from build123d import *

# Parameters (mm, degrees)
SKETCH1_W            = 20
SKETCH1_H            = 20
BOSS_EXTRUDE1_DEPTH  = 6.35
M5_CLEARANCE_HOLE1_D = 5.5
FILLET1_R            = 2.5


with BuildPart() as part:
    # Sketch1 → Boss-Extrude1 (new body)
    with BuildSketch(Plane(origin=(0, 0, 0), x_dir=(1, 0, 0), z_dir=(0, 1, 0))):
        Rectangle(SKETCH1_W, SKETCH1_H)
    extrude(amount=BOSS_EXTRUDE1_DEPTH)

    # M5 Clearance Hole1 (through all)
    with Locations(Plane(origin=(0, 6.35, 0), x_dir=(1, 0, 0), z_dir=(0, 1, 0))):
        with Locations((0, 0)):
            Hole(M5_CLEARANCE_HOLE1_D / 2)

    # Fillet1
    fillet1_edges = [part.edges().sort_by_distance(p)[0] for p in [
        (10, 3.175, 10),
        (-10, 3.175, 10),
        (-10, 3.175, -10),
        (10, 3.175, -10),
    ]]
    fillet(fillet1_edges, radius=FILLET1_R)


solid = part.part
Work out the finished part from the listing and answer in its coordinate system (mm). Coordinates: 2 decimals unless noted, no trailing zeros. Write each loop counter-clockwise with the first axis right and the second up, starting at its lowest first coordinate (ties: lowest second). Pieces come first, ordered by that corner, then holes. Notation, with made-up numbers: M -7.75,-13.75 L 50.25,-13.75 A12 ccw 50.25,-1.75 Z; hole C 32,56 d3. An arc over 180 degrees is marked long. Write item = value, one per line.
1. The part is cut by section B-B (y = 4.25). Determine the outline of the cut face in (x, z).
Solution:
outline = M -10,-7.5 A2.5 ccw -7.5,-10 L 7.5,-10 A2.5 ccw 10,-7.5 L 10,7.5 A2.5 ccw 7.5,10 L -7.5,10 A2.5 ccw -10,7.5 Z; hole C 0,0 d5.5
2. Straight lines are drawn through the part: line 1 (Z direction, x = 0, y = 5); line 2 (Z direction, x = -1.25, y = 1.5); line 3 (X direction, y = 1.25, z = -2.5). For each, find the intervals that lie inside material, in ascending order. Write a range as from..to.
Solution:
line_1 = -10..-2.75, 2.75..10
line_2 = -10..-2.45, 2.45..10
line_3 = -10..-1.15, 1.15..10
3. The part is cut by section C-C (x = 0). Determine the outline of the cut face in (y, z), then the cut area to 3 significant figures.
Solution:
outline = M 0,-10 L 6.35,-10 L 6.35,-2.75 L 0,-2.75 Z; M 0,2.75 L 6.35,2.75 L 6.35,10 L 0,10 Z
area = 92.1 mm2
4. The part is cut by section A-A (z = 0). Determine the outline of the cut face in (x, y), then the cut area to 3 significant figures.
Solution:
outline = M -10,0 L -2.75,0 L -2.75,6.35 L -10,6.35 Z; M 2.75,0 L 10,0 L 10,6.35 L 2.75,6.35 Z
area = 92.1 mm2
